```python
from build123d import *

# Parameters (mm, degrees)
SKETCH_W            = 70
SKETCH_H            = 70
PAD_DEPTH           = 10
SKETCH001_R         = 30.25
SKETCH001_R_2       = 26.85
POCKET_DEPTH        = 5
SKETCH003_R         = 2.25
HOLE_DEPTH          = 10
HOLE_TIPS_R         = 2.25
SKETCH004_R         = 2.25
HOLE001_DEPTH       = 10
HOLE001_TIPS_R      = 2.25
HOLE002_D           = 12
HOLE002_CBORE_D     = 18
HOLE002_CBORE_DEPTH = 7
SKETCH007_R         = 3.3
HOLE003_DEPTH       = 7
HOLE003_TIPS_R      = 3.3


with BuildPart() as part:
    # Sketch → Pad (new body)
    with BuildSketch(Plane.XZ):
        Rectangle(SKETCH_W, SKETCH_H)
    extrude(amount=PAD_DEPTH)

    # Sketch001 (on Face6 of Pad) → Pocket (cut)
    with BuildSketch(Plane.XZ.offset(10)):
        Circle(SKETCH001_R)
        Circle(SKETCH001_R_2, mode=Mode.SUBTRACT)
    extrude(amount=-POCKET_DEPTH, mode=Mode.SUBTRACT)

    # Sketch003 (on Face3 of Pocket) → Hole (cut)
    with BuildSketch(Plane(origin=(35, 0, 0), x_dir=(0, 0, 1), z_dir=(1, 0, 0))):
        with Locations((25, 5)):
            Circle(SKETCH003_R)
    extrude(amount=-HOLE_DEPTH, mode=Mode.SUBTRACT)

    # Hole tips → Hole tip 1 section 0
    with BuildSketch(Plane(origin=(25, 0, 0), x_dir=(0, 0, 1), z_dir=(1, 0, 0)), mode=Mode.PRIVATE) as hole_tip_1_s0:
        with Locations((25, 5)):
            Circle(HOLE_TIPS_R)
    loft([hole_tip_1_s0.sketch, Vertex(23.648064, -5, 25)], mode=Mode.SUBTRACT)

    # Sketch004 (on Face6 of Hole) → Hole001 (cut)
    with BuildSketch(Plane(origin=(0, 0, -35), x_dir=(1, 0, 0), z_dir=(0, 0, -1))):
        with Locations((25, 5)):
            Circle(SKETCH004_R)
    extrude(amount=-HOLE001_DEPTH, mode=Mode.SUBTRACT)

    # Hole001 tips → Hole001 tip 1 section 0
    with BuildSketch(Plane(origin=(0, 0, -25), x_dir=(1, 0, 0), z_dir=(0, 0, -1)), mode=Mode.PRIVATE) as hole001_tip_1_s0:
        with Locations((25, 5)):
            Circle(HOLE001_TIPS_R)
    loft([hole001_tip_1_s0.sketch, Vertex(25, -5, -23.648064)], mode=Mode.SUBTRACT)

    # Hole002 (through all)
    with Locations(Plane(origin=(0, 0, 0), x_dir=(1, 0, 0), z_dir=(0, 1, 0))):
        with Locations((15.33, 0), (0, -15.779452), (0, 15.779452), (-15.33, 0)):
            CounterBoreHole(HOLE002_D / 2, HOLE002_CBORE_D / 2, HOLE002_CBORE_DEPTH)

    # Sketch007 (on Face5 of Hole002) → Hole003 (cut)
    with BuildSketch(Plane.XZ.offset(10)):
        with Locations((14.142136, 14.142136)):
            Circle(SKETCH007_R)
        with Locations((-14.142136, -14.142136)):
            Circle(SKETCH007_R)
    extrude(amount=-HOLE003_DEPTH, mode=Mode.SUBTRACT)

    # Hole003 tips → Hole003 tip 1 section 0
    with BuildSketch(Plane.XZ.offset(3), mode=Mode.PRIVATE) as hole003_tip_1_s0:
        with Locations((14.142136, 14.142136)):
            Circle(HOLE003_TIPS_R)
    loft([hole003_tip_1_s0.sketch, Vertex(14.142136, -1.01716, 14.142136)], mode=Mode.SUBTRACT)

    # Hole003 tips → Hole003 tip 2 section 0
    with BuildSketch(Plane.XZ.offset(3), mode=Mode.PRIVATE) as hole003_tip_2_s0:
        with Locations((-14.142136, -14.142136)):
            Circle(HOLE003_TIPS_R)
    loft([hole003_tip_2_s0.sketch, Vertex(-14.142136, -1.01716, -14.142136)], mode=Mode.SUBTRACT)


solid = part.part
```
Verification items for the finished model (mm, model axes). A direction names the side the tool comes from. Coordinates: 2 decimals unless noted, no trailing zeros. Order: outer loops, then holes, each group sorted by start corner. A loop starts at its lowest first (then second) coordinate and runs counter-clockwise, first axis right, second up. Notation, with made-up numbers: (-28.75, -5.75) -> (17.25, -5.75) arc R20 ccw to (17.25, 28.25) -> close; hole circle Ø6 at (59.5, -29.5). An arc over 180 degrees is marked (long way). Answer as CSV lines item,"result". Start each with the question number.
1) Material ranges on L1, parallel to Z at x = 0, y = -7.15; L2, parallel to Z at x = 0, y = -1.75; L3, parallel to Z at x = 33, y = -5, recorded low to high. Write a range as [from, to].
2) Cross-section at A-A, the plane x = 0. Record the boundary of the cut face in (y, z).
3) Set-up check for faces 5 (the face through (23.914, -3.451, -2.703)), 6 (the face through (-19.79, -7.535, 18.147)), 7 (the face through (-35, -5, 0)): record each of +Z, -Z, +X, -X, +Y, -Y from which the full face is reachable in a straight line by a thin tool's end or side.
4) Release check for a two-part mould opening along Z. For faces 1 (the face through (2, -7, 22)), 2 (the face through (0, -5, -35)), 3 (the face through (0, 0, 0)), 4 (the face through (-10.995, -6.549, -13.151)) record: released by +Z, released by -Z, zero draft, split by the parting line, or undercut.
5) Cross-section at B-B, the plane z = -2. Record the boundary of the cut face in (x, y).
6) Cross-section at C-C, the plane z = -20.5. Record the boundary of the cut face in (x, y), then the cut area to 3 significant figures.
7) Gauge pin test, flat ends, axial feed: pin 1 Ø5.5 at (x, z) = (2.5, -18) entering from +Y; pin 2 Ø3.5 at (y, z) = (-5, 25) entering from +X; pin 3 Ø11 at (x, z) = (-15.33, 0) entering from -Y. Record the tip position at first contact, or that the pin passes through.
Conclusion:
1,L1,"z = [-35, -30.25], [-26.85, -21.78], [-9.78, 9.78], [21.78, 26.85], [30.25, 35]"
1,L2,"z = [-35, -24.78], [-6.78, 6.78], [24.78, 35]"
1,L3,"z = [-35, 22.75], [27.25, 35]"
2,outline,"(-10, -35) -> (0, -35) -> (0, -24.78) -> (-7, -24.78) -> (-7, -21.78) -> (-10, -21.78) -> (-10, -26.85) -> (-5, -26.85) -> (-5, -30.25) -> (-10, -30.25) -> close; (-10, -9.78) -> (-7, -9.78) -> (-7, -6.78) -> (0, -6.78) -> (0, 6.78) -> (-7, 6.78) -> (-7, 9.78) -> (-10, 9.78) -> close; (-10, 21.78) -> (-7, 21.78) -> (-7, 24.78) -> (0, 24.78) -> (0, 35) -> (-10, 35) -> (-10, 30.25) -> (-5, 30.25) -> (-5, 26.85) -> (-10, 26.85) -> close"
3,face 5,"+Y"
3,face 6,"-Y"
3,face 7,"+Z, -Z, -X, +Y, -Y"
4,face 1,"undercut"
4,face 2,"released by -Z"
4,face 3,"zero draft"
4,face 4,"undercut"
5,outline,"(-35, -10) -> (-30.18, -10) -> (-30.18, -5) -> (-26.78, -5) -> (-26.78, -10) -> (-20.99, -10) -> (-20.99, -7) -> (-24.1, -7) -> (-24.1, 0) -> (-35, 0) -> close; (-9.67, -10) -> (9.67, -10) -> (9.67, -7) -> (6.56, -7) -> (6.56, 0) -> (-6.56, 0) -> (-6.56, -7) -> (-9.67, -7) -> close; (20.99, -10) -> (26.78, -10) -> (26.78, -5) -> (30.18, -5) -> (30.18, -10) -> (35, -10) -> (35, 0) -> (24.1, 0) -> (24.1, -7) -> (20.99, -7) -> close"
6,outline,"(-35, -10) -> (-22.24, -10) -> (-22.24, -5) -> (-17.34, -5) -> (-17.34, -10) -> (-3.7, -10) -> (-3.7, -7) -> (-7.66, -7) -> (-7.66, 0) -> (-35, 0) -> close; (3.7, -10) -> (17.34, -10) -> (17.34, -5) -> (22.24, -5) -> (22.24, -10) -> (35, -10) -> (35, 0) -> (7.66, 0) -> (7.66, -7) -> (3.7, -7) -> close"
6,area,"521 mm²"
7,pin 1,"stops at y = -7"
7,pin 2,"stops at x = 24.7"
7,pin 3,"passes through"
